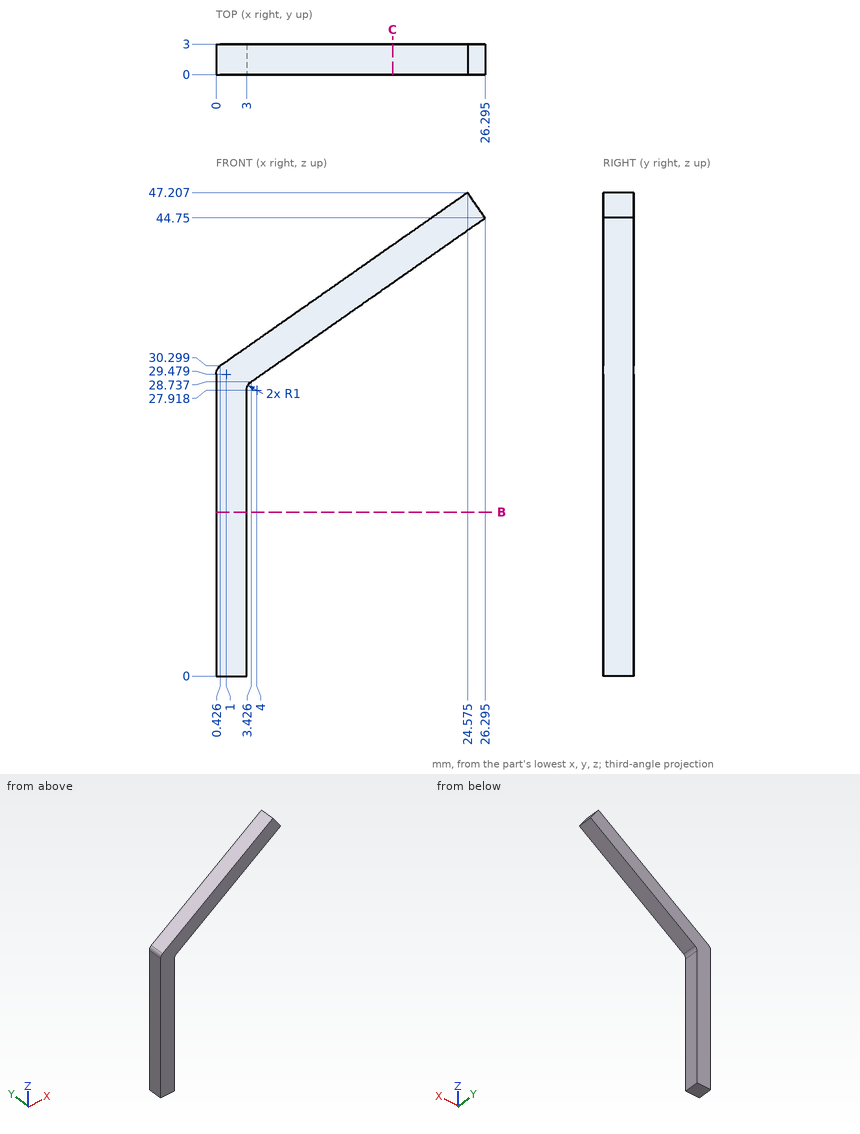
Design review of the part shown in the three views and the two pictorial views. Dimensions are in mm from the part's minimum x, y and z. Give positions to 0.01 mm unless a question says otherwise; leave off trailing zeros. Write each loop counter-clockwise with the first axis right and the second up, starting at its lowest first coordinate (ties: lowest second). Pieces come first, ordered by that corner, then holes.
(1) Add section C-C (x = 17.25). Give the boundary of the cut face in (y, z).
Checked values:
outline: (0, 38.42) - (3, 38.42) - (3, 42.08) - (0, 42.08) - close
(2) Add section B-B (z = 16). Give the boundary of the cut face in (x, y).
Checked values:
outline: (0, 0) - (3, 0) - (3, 3) - (0, 3) - close
(3) Wall thickness on line 1 along X through (y, z) = (0.65, 12.5); line 2 along Z through (x, y) = (20, 1.4) (1 decimal); line 3 along X through (y, z) = (0.1, 33.5): over which ranges is each line inside the solid? List them lowest first.
Checked values:
line 1: x = 0 to 3
line 2: z = 40.3 to 44
line 3: x = 5 to 10.23
(4) Clearance check with flat-ended pins moving along their axes: pin 1 Ø1.5 at (y, z) = (2.5, 38) entering from -X (1 decimal); pin 2 Ø1.5 at (y, z) = (2, 14) entering from +X; pin 3 Ø1 at (x, y) = (9.5, 2.5) entering from -Z. State where each tip first meets the part, or that it passes through.
Checked values:
pin 1: stops at x = 10.4
pin 2: stops at x = 3
pin 3: stops at z = 32.64
